Source: CAD feature listing. Evaluate the final solid. Frame: model axes, mm. Face numbers are marked on the shaded views. Coordinates: 2 decimals unless noted, no trailing zeros. Write each loop counter-clockwise with the first axis right and the second up, starting at its lowest first coordinate (ties: lowest second). Pieces come first, ordered by that corner, then holes. Notation, with made-up numbers: M -3,40.25 L 16,40.25 A16 cw 16,51.25 Z; hole C -8.5,66.5 d3. An arc over 180 degrees is marked long. One line per item, written item: value. Start each with the question number.
Item 1: Cut plane B-B, the plane x = -14. Output: boundary loops of the cut face in (y, z), then the cut area to 3 significant figures.
Item 2: Cut plane D-D, the plane x = 20. Output: boundary loops of the cut face in (y, z), then the cut area to 3 significant figures.
Item 3: Mould query, pull axis Y, two halves, no side actions, for the marked faces 1, 2 and 3. Classes: released by +Y, released by -Y, zero draft, split by the parting line, or undercut.
Item 4: Ray query, L1, parallel to X at y = -1.25, z = 4.6; L2, parallel to X at y = -4.25, z = 4.3; L3, parallel to Y at x = -8.5, z = 0.25. Return the intervals inside material, ascending. Write a range as from..to.
Item 5: Cut plane A-A, the plane y = -4.75. Output: boundary loops of the cut face in (x, z), then the cut area to 3 significant figures.
Item 6: Pin query (flat end, axial travel): P1, Ø9, axis at x = 16.89, y = -0.93, coming from the -Z side; P2, Ø3, axis at y = -6.5, z = 2.5, coming from the +X side. Return the tip coordinate at first contact, or that it passes through.
Item 7: Cut plane C-C, the plane z = 1. Output: boundary loops of the cut face in (x, y), then the cut area to 3 significant figures.
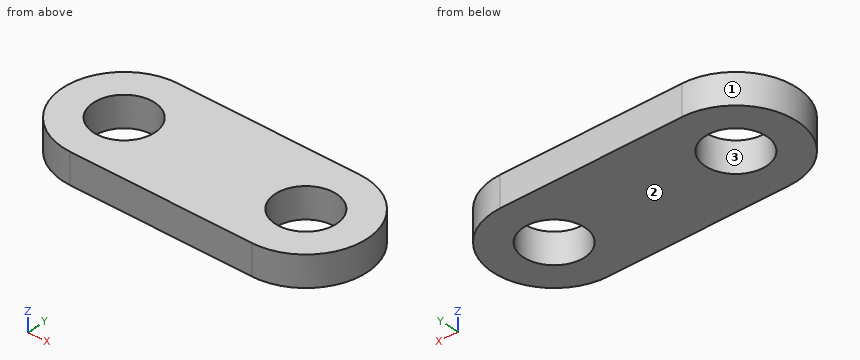
Autodesk Inventor part; units mm, degrees
ref_plane "YZ Plane" through (0, 0, 0) normal (1, 0, 0) x (0, 1, 0)
ref_plane "XZ Plane" through (0, 0, 0) normal (0, 1, 0) x (-1, 0, 0)
ref_plane "XY Plane" through (0, 0, 0) normal (0, 0, 1) x (1, 0, 0)
sketch "Sketch1" plane through (0, 0, 0) normal (0, 0, 1) x (1, 0, 0)
  arc A0 (-13.1138, 9.0719) -> (-13.1138, -10.9281) centre (-13.1138, -0.9281) ccw
  arc A1 (16.8862, -10.9281) -> (16.8862, 9.0719) centre (16.8862, -0.9281) ccw
  line L0 (-13.1138, 9.0719) -> (16.8862, 9.0719)
  line L1 (-13.1138, -10.9281) -> (16.8862, -10.9281)
  circle A2 centre (-13.1138, -0.9281) radius 5
  circle A3 centre (16.8862, -0.9281) radius 5
  point P0 (0, 0)
  dimension "d0" = 20
  dimension "d1" = 20
  dimension "d2" = 30
  dimension "d3" = 10
  dimension "d4" = 10
extrude "Extrusion1" add sketch "Sketch1" along normal blind 5
properties part number "lesson3"
From the geometry:
1. outline: M -10.89,0 L -5.85,0 L -5.85,5 L -10.89,5 Z; M 3.99,0 L 9.03,0 L 9.03,5 L 3.99,5 Z
1. area: 50.4 mm²
2. outline: M -10.43,0 L -4.84,0 L -4.84,5 L -10.43,5 Z; M 2.98,0 L 8.57,0 L 8.57,5 L 2.98,5 Z
2. area: 55.9 mm²
3. face 1: split by the parting line
3. face 2: zero draft
3. face 3: undercut
4. L1: x = -23.11..-18.1, -8.12..11.9, 21.88..26.88
4. L2: x = -22.55..-16.85, -9.38..13.15, 20.62..26.32
4. L3: y = -10.93..-2.85, 1..9.07
5. outline: M -22.35,0 L -16.34,0 L -16.34,5 L -22.35,5 Z; M -9.89,0 L 13.66,0 L 13.66,5 L -9.89,5 Z; M 20.11,0 L 26.13,0 L 26.13,5 L 20.11,5 Z
5. area: 178 mm²
6. P1: passes through
6. P2: stops at x = 26.02
7. outline: M -13.11,-10.93 L 16.89,-10.93 A10 ccw 16.89,9.07 L -13.11,9.07 A10 ccw Z; hole C -13.11,-0.93 d10; hole C 16.89,-0.93 d10
7. area: 757 mm²
